Part print with two shaded views. Sizes in mm from the minimum x, y, z corner. A direction names the side the tool comes from. Round coordinates to 2 decimals unless told otherwise and drop trailing zeros. Write each loop counter-clockwise with the first axis right and the second up, starting at its lowest first coordinate (ties: lowest second). Pieces come first, ordered by that corner, then holes. Notation, with made-up numbers: (52.5, 30) - (57.5, 30) arc R25 ccw to (57.5, 48) - close; hole circle Ø5 at (17, 37). An arc over 180 degrees is marked (long way). Use one line per item in the form item = value. Start each with the question number.
Item 1: Drill centre lines: L1, parallel to Y at x = 7, z = 1.6; L2, parallel to X at y = 1.35, z = 15; L3, parallel to Z at x = 4.75, y = 7.75. Where is each one in solid material? Low to high.
Item 2: Band-saw the part on B-B, the plane x = 8. List the corners of the cut face in (y, z).
Item 3: Band-saw the part on D-D, the plane x = 11.75. List the corners of the cut face in (y, z), and give its area (3 significant figures).
Item 4: Pull direction Z, two halves, no side cores. Call the marked faces 1, 2, 3 and 4: +Z half, -Z half, draft (parallel to the pull), parting line (faces both ways), or undercut.
Item 5: Pin check, flat tips, straight feed: pin 1 (7 mm diameter, centred on x = 10, z = 11, fed in from +Y); pin 2 (1.5 mm diameter, centred on x = 5.5, z = 15, fed in from +Y). Stop position of each tip, or through.
Item 6: Band-saw the part on A-A, the plane z = 15. List the corners of the cut face in (x, y), and give its area (3 significant figures).
Item 7: Tool access for the marked faces 5 and 6: list every direction of +Z, -Z, +X, -X, +Y, -Y with a clear straight run to the whole face (end or side of a thin tool).
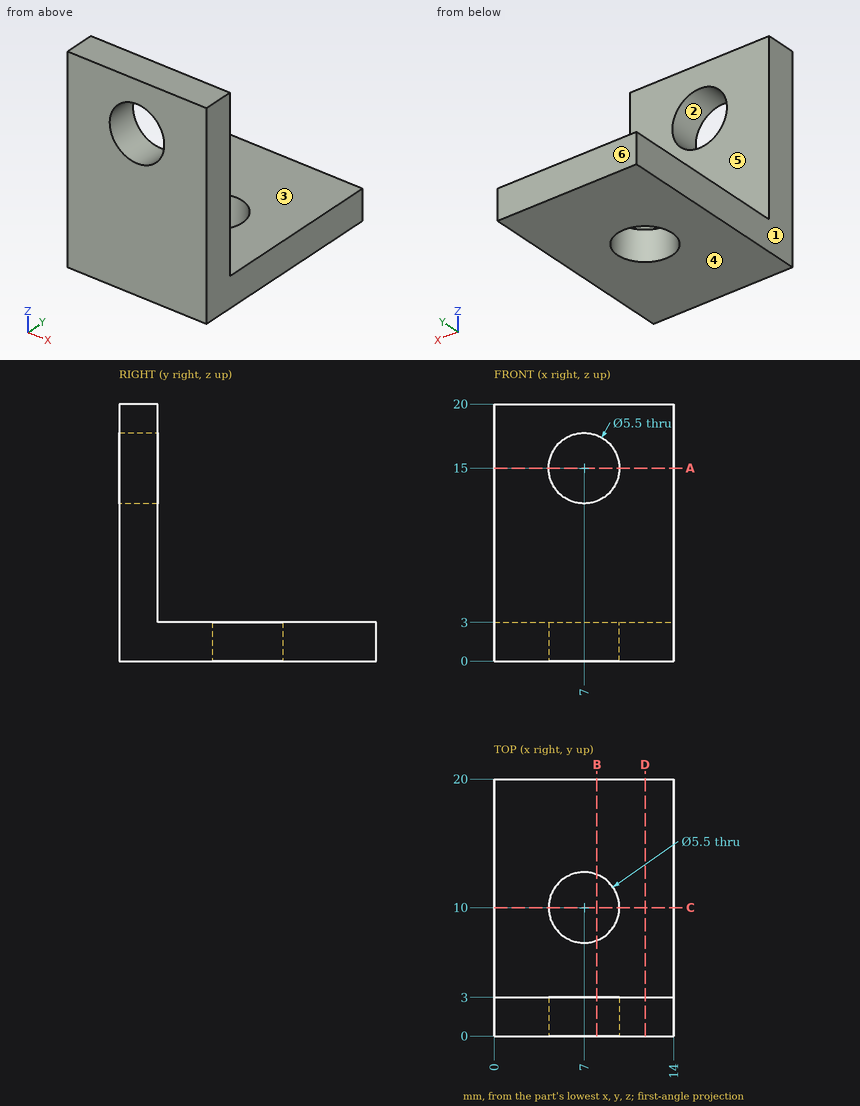
Determined:
q1.L1 = 0 to 7.25, 12.75 to 20
q1.L2 = 0 to 4.25, 9.75 to 14
q1.L3 = 0 to 3
q2.outline = (0, 0) - (7.44, 0) - (7.44, 3) - (3, 3) - (3, 12.44) - (0, 12.44) - close; (0, 17.56) - (3, 17.56) - (3, 20) - (0, 20) - close; (12.56, 0) - (20, 0) - (20, 3) - (12.56, 3) - close
q3.outline = (0, 0) - (20, 0) - (20, 3) - (3, 3) - (3, 20) - (0, 20) - close
q3.area = 111 mm²
q4.face_1 = draft
q4.face_2 = undercut
q4.face_3 = +Z half
q4.face_4 = -Z half
q5.pin_1 = 3
q5.pin_2 = through
q6.outline = (0, 0) - (4.25, 0) - (4.25, 3) - (0, 3) - close; (9.75, 0) - (14, 0) - (14, 3) - (9.75, 3) - close
q6.area = 25.5 mm²
q7.face_5 = +Z, +X, -X, +Y
q7.face_6 = +Z, -Z, +X, -X, +Y
